Geometry: see drawing. Coordinates: mm, zero at the bounding-box minimum. A direction names the side the tool comes from. Coordinates: 2 decimals unless noted, no trailing zeros. Order: outer loops, then holes, each group sorted by start corner. A loop starts at its lowest first (then second) coordinate and runs counter-clockwise, first axis right, second up.
Item 1: Mould query, pull axis X, two halves, no side actions, for the marked faces 3, 4 and 5. Classes: released by +X, released by -X, zero draft, split by the parting line, or undercut.
Item 2: Section C-C on z = 30. Return the cut outline in (x, y) (3 decimals), then the cut area to 3 significant figures.
Item 3: Contact query for flat-ended pins moving along their axis: P1, Ø5, axis at y = 20.5, z = 46.5, coming from the -X side; P2, Ø1.9, axis at x = 13.5, y = 11.5, coming from the +Z side; P3, Ø4, axis at x = 12.7, y = 12.7, coming from the -Z side. Output: stop coordinate, or through.
Item 4: Ray query, line 1 (Y direction, x = 12.7, z = 10.25); line 2 (Z direction, x = 4.75, y = 16.25); line 3 (Y direction, x = 15.75, z = 20.5). Return the intervals inside material, ascending.
Item 5: Reachability of the marked faces 1 and 2 from +Z, -Z, +X, -X, +Y, -Y: full face, straight path, thin tool, end or side. Return the list, or none.
Item 6: Section A-A on x = 12.7. Return the cut outline in (y, z) (3 decimals), then the cut area to 3 significant figures.
Item 7: Section D-D on x = 18.25. Return the cut outline in (y, z).
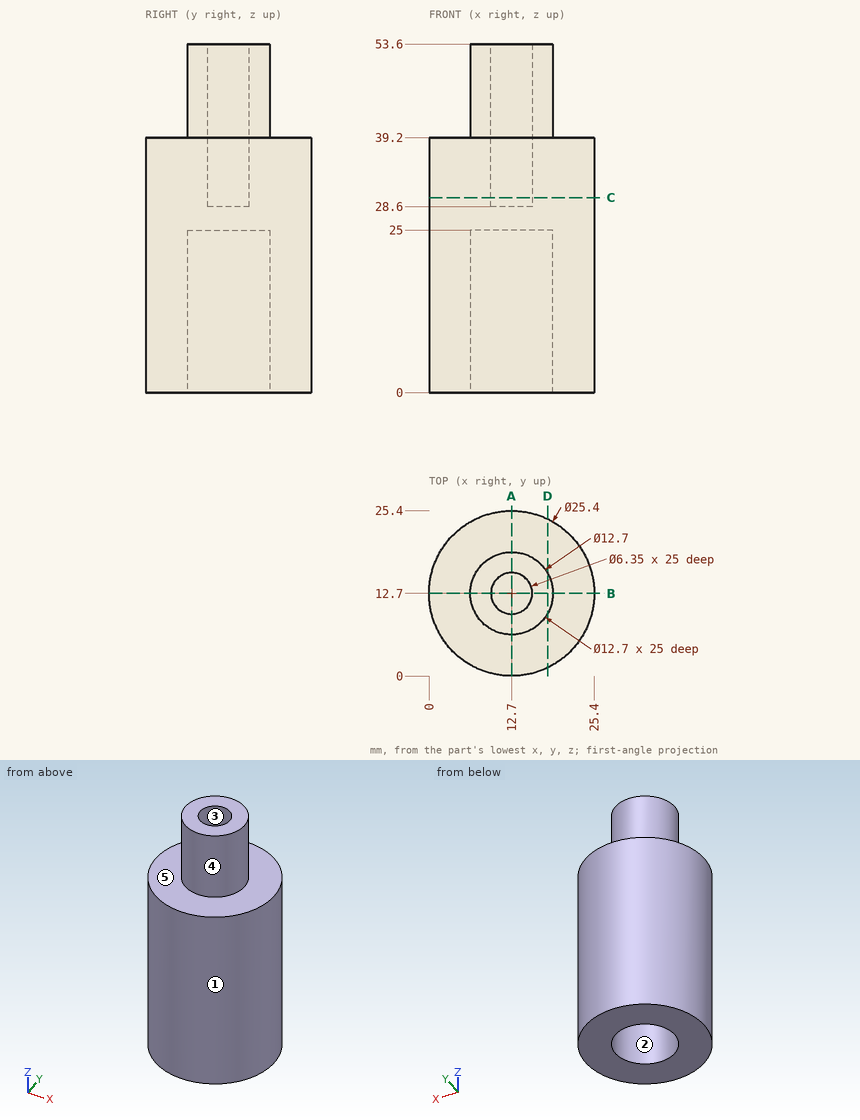
Answer list:
1. face 3: undercut
1. face 4: split by the parting line
1. face 5: zero draft
2. outline: circle Ø25.4 at (12.7, 12.7); hole circle Ø6.35 at (12.7, 12.7)
2. area: 475 mm2
3. P1: stops at x = 9.2
3. P2: stops at z = 28.6
3. P3: stops at z = 25
4. line 1: y = 0 to 6.35, 19.05 to 25.4
4. line 2: z = 0 to 39.2
4. line 3: y = 0.37 to 7.13, 18.27 to 25.03
5. face 1: +Z, -Z
5. face 2: -Z
6. outline: (0, 0) - (6.35, 0) - (6.35, 25) - (19.05, 25) - (19.05, 0) - (25.4, 0) - (25.4, 39.2) - (19.05, 39.2) - (19.05, 53.6) - (15.875, 53.6) - (15.875, 28.6) - (9.525, 28.6) - (9.525, 53.6) - (6.35, 53.6) - (6.35, 39.2) - (0, 39.2) - close
6. area: 702 mm2
7. outline: (1.28, 0) - (9.61, 0) - (9.61, 25) - (15.79, 25) - (15.79, 0) - (24.12, 0) - (24.12, 39.2) - (15.79, 39.2) - (15.79, 53.6) - (9.61, 53.6) - (9.61, 39.2) - (1.28, 39.2) - close
